Verification items for the finished model (mm, model axes). Face numbers are marked on the shaded views. A direction names the side the tool comes from. Coordinates: 2 decimals unless noted, no trailing zeros. Order: outer loops, then holes, each group sorted by start corner. A loop starts at its lowest first (then second) coordinate and runs counter-clockwise, first axis right, second up. Notation, with made-up numbers: M 54.25,40 L 93.25,40 A27 ccw 93.25,76 Z; hole C 14,58.25 d2. An arc over 180 degrees is marked long. Write item = value, one per line.
Solid Edge part; units mm, degrees
sketch "Sketch1" plane through (0, 0, 0) normal (0, 0, 1) x (1, 0, 0)
  line L0 (-11.4, -6.15) -> (11.4, -6.15)
  line L1 (11.4, -6.15) -> (11.4, 6.15)
  line L2 (11.4, 6.15) -> (-11.4, 6.15)
  line L3 (-11.4, 6.15) -> (-11.4, -6.15)
  dimension "D1" = 11.4
  dimension "D2" = 11.4
extrude "Protrusion1" add sketch "Sketch1" along normal blind 22.4
sketch "Sketch2" plane through (0, 0, 22.4) normal (0, 0, 1) x (1, 0, 0)
  arc A0 (0.2256, 2.8) -> (0.2256, -2.8) centre (-5.25, 0) ccw
  line L0 (0.2256, -2.8) -> (0.6, -2.8)
  arc A1 (0.6, 2.8) -> (0.6, -2.8) centre (0.6, 0) cw
  line L1 (0.2256, 2.8) -> (0.6, 2.8)
  dimension "D1" = 0.2256
extrude "Extrusionsausprägung_2" add sketch "Sketch2" along normal blind 6
sketch "Sketch3" plane through (-4, 0, 28.4) normal (0, 0, 1) x (1, 0, 0)
  circle A0 centre (-1.25, 0) radius 2.4
extrude "Extrusionsausprägung_3" add sketch "Sketch3" along normal blind 4.4
sketch "Sketch4" plane through (-11.4, 0, 11.35) normal (-1, 0, 0) x (0, 0, 1)
  circle A0 centre (-6.35, -1.3) radius 0.6
  circle A1 centre (-6.35, 0) radius 0.6
  circle A2 centre (-6.35, 1.3) radius 0.6
  dimension "D1" = 6.35
extrude "Extrusionsausprägung_4" add sketch "Sketch4" along normal blind 3
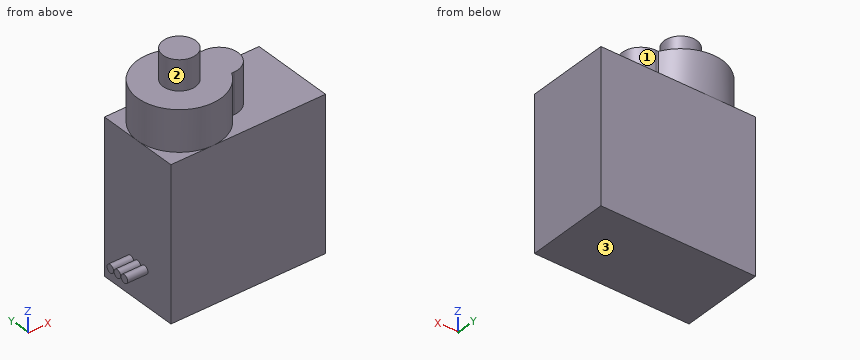
Item 1: Scan lines: L1, parallel to X at y = 3.25, z = 8; L2, parallel to Z at x = 6.5, y = 3.5; L3, parallel to Z at x = -5.5, y = 5.5. Record each from-to range of solid material in increasing order. Write a range as from..to.
Report:
L1 = -11.4..11.4
L2 = 0..22.4
L3 = 0..28.4
Item 2: Sectioned sample at C-C, the plane x = -10. Enter the section's corners in (y, z).
Report:
outline = M -6.15,0 L 6.15,0 L 6.15,22.4 L 3.91,22.4 L 3.91,28.4 L -3.91,28.4 L -3.91,22.4 L -6.15,22.4 Z
Item 3: Tool access check on the marked faces 1, 2 and 3. Record the directions out of +Z, -Z, +X, -X, +Y, -Y that give a thin tool (end or side, any length) a straight path to the whole face; none if there is none.
Report:
face_1 = +Z, +X
face_2 = +Z
face_3 = -Z, +X, -X, +Y, -Y
Item 4: Gauge pin test, flat ends, axial feed: pin 1 (1.5 mm diameter, centred on y = 2, z = 14, fed in from -X); pin 2 (2 mm diameter, centred on y = 1, z = 27.5, fed in from +X); pin 3 (3 mm diameter, centred on x = -9, y = 4, fed in from +Z). Record the tip position at first contact, or that the pin passes through.
Report:
pin_1 = -11.4
pin_2 = 3.4
pin_3 = 28.4
Item 5: Sectioned sample at B-B, the plane y = -3.25. Enter the section's corners in (x, z).
Report:
outline = M -11.4,0 L 11.4,0 L 11.4,22.4 L -0.03,22.4 L -0.03,28.4 L -10.47,28.4 L -10.47,22.4 L -11.4,22.4 Z
Item 6: Sectioned sample at A-A, the plane z = 5. Enter the section's corners in (x, y), then the cut area to 3 significant figures.
Report:
outline = M -14.4,-1.9 L -11.4,-1.9 L -11.4,-6.15 L 11.4,-6.15 L 11.4,6.15 L -11.4,6.15 L -11.4,1.9 L -14.4,1.9 L -14.4,0.7 L -11.4,0.7 L -11.4,0.6 L -14.4,0.6 L -14.4,-0.6 L -11.4,-0.6 L -11.4,-0.7 L -14.4,-0.7 Z
area = 291 mm^2
Item 7: Sectioned sample at D-D, the plane z = 24. Enter the section's corners in (x, y).
Report:
outline = M 0.23,-2.8 L 0.6,-2.8 A2.8 ccw 0.6,2.8 L 0.23,2.8 A6.15 ccw long Z
